```python
from build123d import *

# Parameters (mm, degrees)
F0_W     = 99
F0_H     = 50
F1_DEPTH = 5
F3_DEPTH = 127
F5_DEPTH = 152.4


with BuildPart() as f1:
    # F0 (on Top) → F1 (new body)
    with BuildSketch(Plane.XY):
        Rectangle(F0_W, F0_H)
    extrude(amount=F1_DEPTH)

    # F2 (on face) → F3 (cut)
    with BuildSketch(Plane.YZ.offset(49.5)):
        Polygon((-21.321116, 2.410467), (0, 5), (-25, 5), (-25, 0), align=None)
    extrude(amount=-F3_DEPTH, mode=Mode.SUBTRACT)

    # F4 (on face) → F5 (cut)
    with BuildSketch(Plane.YZ.offset(49.5)):
        Polygon((25, 2.5), (-10.516109, 0), (25, 0), align=None)
    extrude(amount=-F5_DEPTH, mode=Mode.SUBTRACT)


solid = f1.part
```
Can you work these out from the model? Positions are in its coordinate system, mm. Coordinates: 2 decimals unless noted, no trailing zeros. Loops run counter-clockwise (first coordinate to the right, second up) from the corner with the lowest first, then second, coordinate; pieces in that order, holes last. Notation, with made-up numbers: (54.25, 40.5) -> (68.25, 40.5) arc R31 ccw to (68.25, 73.5) -> close; hole circle Ø10 at (80.5, 67.5). An arc over 180 degrees is marked (long way). Put each result on its own line as item: value. Start each with the question number.
Q1. I want a section at A-A (x = 11). Write out the boundary of the cut face in (y, z).
Q2. I want a section at C-C (z = 3.8). Write out the boundary of the cut face in (x, y), plus the area to 3 significant figures.
Q3. If I drill on line 1 (Z direction, x = -14, y = 7); line 2 (Z direction, x = -9.5, y = 18.5), over which ranges is the centre line in solid material (lowest first)? Write a range as [from, to].
Q4. I want a section at B-B (y = -12). Write out the boundary of the cut face in (x, z).
Taken from the geometry:
1. outline: (-25, 0) -> (-10.52, 0) -> (25, 2.5) -> (25, 5) -> (0, 5) -> (-21.32, 2.41) -> close
2. outline: (-49.5, -9.88) -> (49.5, -9.88) -> (49.5, 25) -> (-49.5, 25) -> close
2. area: 3,450 mm2
3. line 1: z = [1.23, 5]
3. line 2: z = [2.04, 5]
4. outline: (-49.5, 0) -> (49.5, 0) -> (49.5, 3.54) -> (-49.5, 3.54) -> close
